The drawing under review shows one solid part. Ordinate dimensions are in mm from its lowest x, y, z. A direction names the side the tool comes from. Coordinates: 2 decimals unless noted, no trailing zeros. Write each loop counter-clockwise with the first axis right and the second up, starting at its lowest first coordinate (ties: lowest second). Pieces come first, ordered by that corner, then holes.
Q1. For probe 1 along X at (y, z) = (62, 30); probe 2 along X at (y, z) = (29, 30); probe 3 along Y at (x, z) = (156.5, 23), list the stretches that pass through material, from the lowest coordinate up.
Q2. Take a section at C-C (z = 18). State how many separate pieces and enclosed holes the cut face has, and give its area (3 significant figures).
Q3. Machinability: for the marked faces 4, 5, 6, 7 and 8, which of the approach directions +Z, -Z, +X, -X, +Y, -Y give a long, thin tool a straight path to every point of the face, cutting with its end or side? Answer none if there is none.
Q4. Take a section at B-B (x = 135). Give the boundary of the cut face in (y, z).
Q5. Mouldability with a two-part tool opening along Z and no side actions: class the marked faces 1, 2 and 3 as pulls with the +Z half, pulls with the -Z half, needs draft (parallel to the pull), parting line crosses it, or undercut.
Q6. Take a section at D-D (z = 47). Give the boundary of the cut face in (x, y).
Q7. Insertion check: pin 1 (18.5 mm diameter, centred on x = 65, y = 37, fed in from +Z); pin 2 (24 mm diameter, centred on x = 25, z = 30, fed in from -Y); pin 3 (18 mm diameter, centred on y = 60, z = 20.5, fed in from -X); pin 4 (15 mm diameter, centred on x = 63.5, z = 23, fed in from +Y). Each pin has a flat end and moves straight along its axis. Give the tip position at first contact, or say it passes through.
Q8. Take a section at A-A (y = 14.5). Give the boundary of the cut face in (x, z), and give its area (3 significant figures).
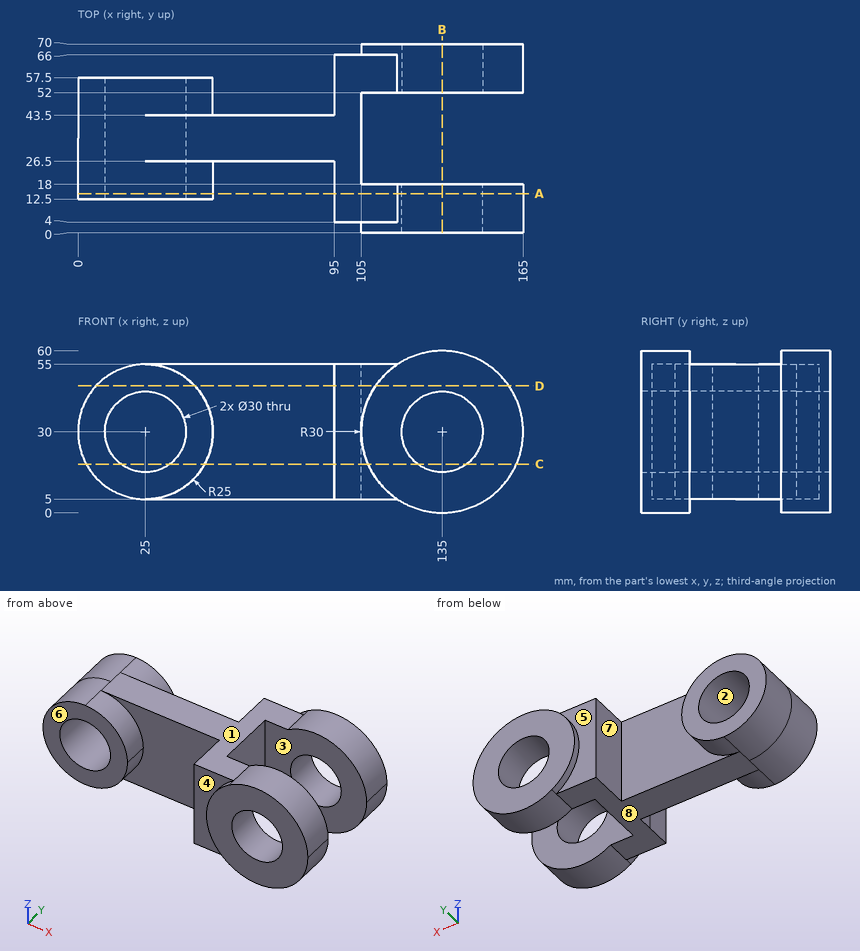
Response:
1. probe 1: x = 95 to 120, 150 to 165
1. probe 2: x = 0 to 10, 40 to 105
1. probe 3: y = 0 to 18, 52 to 70
2. separate pieces: 4
2. enclosed holes: 0
2. area: 4,000 mm2
3. face 4: -X, -Y
3. face 5: -X, +Y
3. face 6: +Z, -Z, -X, -Y
3. face 7: +Z, -Z, +Y
3. face 8: -Z, -X, +Y, -Y
4. outline: (0, 0) - (18, 0) - (18, 15) - (0, 15) - close; (0, 45) - (18, 45) - (18, 60) - (0, 60) - close; (52, 0) - (70, 0) - (70, 15) - (52, 15) - close; (52, 45) - (70, 45) - (70, 60) - (52, 60) - close
5. face 1: pulls with the +Z half
5. face 2: undercut
5. face 3: needs draft
6. outline: (6.67, 12.5) - (43.33, 12.5) - (43.33, 26.5) - (95, 26.5) - (95, 4) - (110.28, 4) - (110.28, 0) - (159.72, 0) - (159.72, 18) - (105, 18) - (105, 52) - (159.72, 52) - (159.72, 70) - (110.28, 70) - (110.28, 66) - (95, 66) - (95, 43.5) - (43.33, 43.5) - (43.33, 57.5) - (6.67, 57.5) - close
7. pin 1: stops at z = 55
7. pin 2: passes through
7. pin 3: stops at x = 0.01
7. pin 4: stops at y = 43.5
8. outline: circle Ø50 at (25, 30); (95, 5) - (118.42, 5) arc R30 ccw (long way) to (118.42, 55) - (95, 55) - close; hole circle Ø30 at (25, 30); hole circle Ø30 at (135, 30)
8. area: 4,080 mm2
